Geometry check sheet. Reference: the model listing, model coordinates, mm. Give positions to 0.01 mm unless a question says otherwise; leave off trailing zeros. Loops run counter-clockwise (first coordinate to the right, second up) from the corner with the lowest first, then second, coordinate; pieces in that order, holes last. Notation, with made-up numbers: (32, -12.75) -> (55, -12.75) arc R23 ccw to (55, 13.25) -> close; hole circle Ø8 at (-1, -5.5). An arc over 180 degrees is marked (long way). One line per item, written item: value. Start each with the question number.
(1) Sectioned sample at A-A, the plane y = 0. Record the cut outline in (x, z).
(2) Draft check along X on faces 1 (the face through (-0.867, 3.905, 3.204)), 2 (the face through (-0.04, -7.41, 6.34)), 3 (the face through (-3.451, 6.033, 3.204)). Enter one of: pulls with the +X half, pulls with the -X half, needs draft (parallel to the pull), parting line crosses it, or undercut.
(3) Sectioned sample at B-B, the plane z = 2.5. Record the cut outline in (x, y).
(4) Scan lines: line 1 along X through (y, z) = (0, 4.5); line 2 along Y through (x, z) = (3.25, 1.5); line 3 along Y through (x, z) = (0, 0.5). Record each from-to range of solid material in increasing order. Write a range as from..to.
(5) Sectioned sample at C-C, the plane x = 3.25. Record the cut outline in (y, z).
(6) Gauge pin test, flat end, axial feed: pin 1 Ø7 at (x, y) = (0, 0) entering from +Z. Record the tip position at first contact, or that the pin passes through.
from build123d import *

# Parameters (mm, degrees)
F0_R     = 4
F1_DEPTH = 15
F3_DEPTH = 6.5
F7_R     = 4
F8_DEPTH = 21.5


with BuildPart() as f1:
    # F0 (on Top) → F1 (new body)
    with BuildSketch(Plane.XY):
        Circle(F0_R)
    extrude(amount=-F1_DEPTH)

    # F2 (on Top) → F3 (join)
    with BuildSketch(Plane.XY):
        Polygon((7, 3.984384), (0, 8.025836), (-7, 3.984384), (-7, -4.098519), (0, -8.139971), (7, -4.098519), align=None)
    extrude(amount=F3_DEPTH)

    # F6: sweep along a path in F5
    with BuildLine(Plane.XY.offset(6.5)) as f6_path:
        CenterArc((0, 0), 8.139971, 0, 360)
    # F4 (on Right) → F6 (sweep, cut)
    with BuildSketch(Plane.YZ):
        Polygon((-8.139971, 5.9), (-7.139971, 6.5), (-8.139971, 6.5), align=None)
        Polygon((-7.139971, 0), (-8.139971, 0.6), (-8.139971, 0), align=None)
    sweep(path=f6_path.line, mode=Mode.SUBTRACT)

    # F7 (on face) → F8 (cut, through all)
    with BuildSketch(Plane(origin=(0, 0, -15), x_dir=(1, 0, 0), z_dir=(0, 0, -1))):
        Circle(F7_R)
    extrude(amount=-F8_DEPTH, mode=Mode.SUBTRACT)


solid = f1.part
Calculated:
1. outline: (-7, 0) -> (-4, 0) -> (-4, 6.5) -> (-7, 6.5) -> close; (4, 0) -> (7, 0) -> (7, 6.5) -> (4, 6.5) -> close
2. face 1: undercut
2. face 2: parting line crosses it
2. face 3: pulls with the -X half
3. outline: (-7, -4.1) -> (0, -8.14) -> (7, -4.1) -> (7, 3.98) -> (0, 8.03) -> (-7, 3.98) -> close; hole circle Ø8 at (0, 0)
4. line 1: x = -7..-4, 4..7
4. line 2: y = -6.26..-2.33, 2.33..6.15
4. line 3: y = -7.97..-4, 4..7.97
5. outline: (-6.26, 0) -> (-2.33, 0) -> (-2.33, 6.5) -> (-6.26, 6.5) -> close; (2.33, 0) -> (6.15, 0) -> (6.15, 6.5) -> (2.33, 6.5) -> close
6. pin 1: passes through
